from build123d import *

# Parameters (mm, degrees)
SKETCH1_W           = 7
SKETCH1_H           = 7
BOSS_EXTRUDE1_DEPTH = 3
CUT_EXTRUDE1_DEPTH  = 7
CUT_EXTRUDE2_DEPTH  = 11
SKETCH4_R           = 1.8
CUT_EXTRUDE3_DEPTH  = 0.8
CUT_EXTRUDE4_DEPTH  = 0.4


with BuildPart() as part:
    # Sketch1 → Boss-Extrude1 (new body)
    with BuildSketch(Plane(origin=(0, 0, 0), x_dir=(1, 0, 0), z_dir=(0, 1, 0))):
        with Locations((3.5, 3.5)):
            Rectangle(SKETCH1_W, SKETCH1_H)
    extrude(amount=BOSS_EXTRUDE1_DEPTH)

    # Sketch2 → Cut-Extrude1 (cut)
    with BuildSketch(Plane.XY):
        Polygon((0, 0), (0.7, 3), (0, 3), align=None)
        Polygon((7, 0), (6.3, 3), (7, 3), align=None)
    extrude(amount=-CUT_EXTRUDE1_DEPTH, mode=Mode.SUBTRACT)

    # Sketch3 → Cut-Extrude2 (cut)
    with BuildSketch(Plane(origin=(0, 0, 0), x_dir=(0, 0, -1), z_dir=(1, 0, 0))):
        Polygon((0, 0), (0.7, 3), (0, 3), align=None)
        Polygon((7, 3), (6.3, 3), (7, 0), align=None)
    extrude(amount=CUT_EXTRUDE2_DEPTH, mode=Mode.SUBTRACT)

    # Sketch4 → Cut-Extrude3 (cut)
    with BuildSketch(Plane.XZ):
        with Locations(Location((3.5, -3.5, 0), (0, 0, 270))):
            Circle(SKETCH4_R)
    extrude(amount=-CUT_EXTRUDE3_DEPTH, mode=Mode.SUBTRACT)

    # Sketch5 → Cut-Extrude4 (cut)
    with BuildSketch(Plane(origin=(0, 3, 0), x_dir=(1, 0, 0), z_dir=(0, 1, 0))):
        with BuildLine():
            Line((2.046721013, 2.878720245), (2.719797936, 2.92359204))
            add(Edge.make_bspline(
                [(2.719797936, 2.92359204), (2.725160149, 2.895432871), (2.735575908, 2.840735478), (2.758717767, 2.762784225), (2.784190549, 2.69011155), (2.81463192, 2.623496744), (2.847957445, 2.561708471), (2.886904829, 2.506506929), (2.928757004, 2.456129675), (2.975585733, 2.412386043), (3.026605026, 2.374074766), (3.082069463, 2.341401632), (3.14137804, 2.313122445), (3.204675773, 2.289835431), (3.272615043, 2.272451562), (3.344603998, 2.260083969), (3.420745884, 2.252164104), (3.4727828, 2.251073777), (3.499445372, 2.250515117)],
                knots=[0, 0, 0, 0, 1.204560339, 2.339781841, 3.415289417, 4.440034832, 5.416475564, 6.362424008, 7.275913008, 8.16578645, 9.05021719, 9.95355393, 10.867835453, 11.809845306, 12.784702352, 13.812224031, 14.87903166, 16, 16, 16, 16], degree=3))
            add(Edge.make_bspline(
                [(3.499445372, 2.250515117), (3.527509416, 2.250821294), (3.582095427, 2.251416824), (3.661196592, 2.258804896), (3.735159775, 2.269389104), (3.803331854, 2.286143658), (3.866985877, 2.304880975), (3.924540945, 2.330515622), (3.976928433, 2.36008148), (4.024013382, 2.393631069), (4.06510446, 2.430839971), (4.101052986, 2.469684857), (4.132361778, 2.5093265), (4.157004013, 2.551524023), (4.176946643, 2.594570783), (4.190127325, 2.639750939), (4.199031656, 2.686027058), (4.200052723, 2.717653631), (4.200567167, 2.733588033)],
                knots=[0, 0, 0, 0, 1.417779877, 2.757654889, 4.012140507, 5.189587551, 6.302846416, 7.360586765, 8.365575446, 9.33904572, 10.275781718, 11.161696098, 12.012180333, 12.822428111, 13.625933072, 14.403138519, 15.195454004, 16, 16, 16, 16], degree=3))
            add(Edge.make_bspline(
                [(4.200567167, 2.733588033), (4.199936245, 2.753552546), (4.198701939, 2.792610195), (4.183842132, 2.848447381), (4.161557458, 2.900178921), (4.12800444, 2.94704074), (4.082900924, 2.989865612), (4.025366896, 3.029927231), (3.953796381, 3.065967021), (3.900700369, 3.086070082), (3.872442167, 3.096769123)],
                knots=[0, 0, 0, 0, 0.90494901, 1.770400303, 2.607161909, 3.452839393, 4.36912122, 5.420987164, 6.627424851, 8, 8, 8, 8], degree=3))
            add(Edge.make_bspline(
                [(3.872442167, 3.096769123), (3.860317321, 3.100832215), (3.833183883, 3.109924755), (3.786897121, 3.12292623), (3.731143485, 3.139161617), (3.665117302, 3.157615727), (3.588840772, 3.176489423), (3.503165804, 3.199739676), (3.407047926, 3.222875577), (3.339803742, 3.239954494), (3.304533513, 3.248912553)],
                knots=[0, 0, 0, 0, 0.521821638, 1.167752076, 1.961721917, 2.891982557, 3.96540661, 5.168436773, 6.514817513, 8, 8, 8, 8], degree=3))
            add(Edge.make_bspline(
                [(3.304533513, 3.248912553), (3.258601207, 3.260380777), (3.169982333, 3.282506842), (3.043591527, 3.321867543), (2.927183282, 3.360974579), (2.821878423, 3.403407811), (2.726515392, 3.446291426), (2.642636716, 3.492636137), (2.568492031, 3.540035098), (2.525286202, 3.57546224), (2.504553545, 3.592462232)],
                knots=[0, 0, 0, 0, 1.293880989, 2.496331788, 3.617634808, 4.64976062, 5.598842568, 6.473791081, 7.267636666, 8, 8, 8, 8], degree=3))
            add(Edge.make_bspline(
                [(2.504553545, 3.592462232), (2.478842356, 3.616535508), (2.428433193, 3.663733391), (2.362077353, 3.741288571), (2.306320379, 3.82321321), (2.260426285, 3.908902595), (2.225088701, 3.998850035), (2.200041876, 4.092453462), (2.18383066, 4.189957168), (2.182176417, 4.256359502), (2.181336398, 4.290078418)],
                knots=[0, 0, 0, 0, 1.064429417, 2.086912298, 3.078678339, 4.055528992, 5.020032834, 5.993708893, 6.981211098, 8, 8, 8, 8], degree=3))
            add(Edge.make_bspline(
                [(2.181336398, 4.290078418), (2.182972343, 4.333710293), (2.18621757, 4.420262908), (2.215978417, 4.547483438), (2.262337684, 4.670241451), (2.316103441, 4.767715859), (2.367760734, 4.841455617), (2.410658355, 4.894370593), (2.457785536, 4.943893923), (2.509787819, 4.988817578), (2.564734232, 5.031772991), (2.624753609, 5.069917913), (2.688144219, 5.105848319), (2.779877653, 5.148442144), (2.904426487, 5.192829094), (3.06647121, 5.230244475), (3.242905826, 5.252735952), (3.365228488, 5.25549518), (3.428632071, 5.256925373)],
                knots=[0, 0, 0, 0, 1.180131776, 2.341029169, 3.518901375, 4.725685298, 5.343762192, 5.955650671, 6.568945152, 7.192346361, 7.815201106, 8.455999361, 9.116257477, 9.787318263, 11.192748436, 12.688084276, 14.283332633, 16, 16, 16, 16], degree=3))
            add(Edge.make_bspline(
                [(3.428632071, 5.256925373), (3.480546978, 5.25623114), (3.581520363, 5.254880873), (3.727893013, 5.241226755), (3.86461301, 5.219975735), (3.991200587, 5.189469994), (4.107714725, 5.149163904), (4.214607068, 5.10115173), (4.311786782, 5.044149232), (4.3980708, 4.977829293), (4.474941591, 4.904715813), (4.541999061, 4.824854673), (4.599499587, 4.739254471), (4.647814268, 4.647977762), (4.68575566, 4.550555251), (4.713622114, 4.447108501), (4.732053229, 4.337881002), (4.736673044, 4.263037228), (4.739028705, 4.224874091)],
                knots=[0, 0, 0, 0, 1.325124071, 2.577337985, 3.749592149, 4.855247722, 5.896868755, 6.892903601, 7.842551483, 8.766257401, 9.665194363, 10.546067736, 11.423174165, 12.293291263, 13.177512979, 14.086532529, 15.024315359, 16, 16, 16, 16], degree=3))
            Line((4.739028705, 4.224874091), (4.065951782, 4.180002296))
            add(Edge.make_bspline(
                [(4.065951782, 4.180002296), (4.062068972, 4.201108183), (4.054501777, 4.242241362), (4.038048624, 4.301152432), (4.019490266, 4.355638451), (3.997768669, 4.405699072), (3.971531605, 4.45043766), (3.942978139, 4.491261716), (3.911320612, 4.527627281), (3.875510829, 4.55853855), (3.83677937, 4.586666537), (3.792639157, 4.60921177), (3.744939713, 4.630128784), (3.691866364, 4.645853249), (3.634438311, 4.65832646), (3.572622102, 4.667573288), (3.506289601, 4.672088109), (3.460655286, 4.673079253), (3.437045532, 4.67359204)],
                knots=[0, 0, 0, 0, 1.151066407, 2.24330871, 3.278475654, 4.238599069, 5.165719782, 6.056502506, 6.909492653, 7.744782051, 8.590364415, 9.471203867, 10.39832458, 11.382154319, 12.435022857, 13.550631277, 14.73277401, 16, 16, 16, 16], degree=3))
            add(Edge.make_bspline(
                [(3.437045532, 4.67359204), (3.412497837, 4.673139334), (3.364739198, 4.672258574), (3.295142133, 4.666853479), (3.229854863, 4.656876194), (3.168556746, 4.643888244), (3.11132966, 4.626219037), (3.058294374, 4.604674333), (3.009208245, 4.579309585), (2.979277664, 4.559353476), (2.964489443, 4.549493482)],
                knots=[0, 0, 0, 0, 1.186678824, 2.308736671, 3.37120409, 4.377216403, 5.334874112, 6.262130804, 7.141346615, 8, 8, 8, 8], degree=3))
            add(Edge.make_bspline(
                [(2.964489443, 4.549493482), (2.947565565, 4.53602445), (2.914789266, 4.509939115), (2.879515034, 4.458142509), (2.858279864, 4.399639797), (2.855723971, 4.358268553), (2.854413321, 4.337053578)],
                knots=[0, 0, 0, 0, 1.037857257, 2.010007357, 2.979541333, 4, 4, 4, 4], degree=3))
            add(Edge.make_bspline(
                [(2.854413321, 4.337053578), (2.855485194, 4.317226776), (2.857596612, 4.27817113), (2.878892988, 4.22269174), (2.911643913, 4.171286094), (2.942244281, 4.143361874), (2.958179346, 4.128820405)],
                knots=[0, 0, 0, 0, 0.98538058, 1.941042925, 2.927803204, 4, 4, 4, 4], degree=3))
            add(Edge.make_bspline(
                [(2.958179346, 4.128820405), (2.970825874, 4.119382262), (2.9990856, 4.098291942), (3.050851816, 4.07148415), (3.113334997, 4.042449691), (3.187959609, 4.014065302), (3.274229699, 3.985733602), (3.372150512, 3.956152032), (3.481782274, 3.926173301), (3.600330525, 3.897140369), (3.720690389, 3.868602665), (3.835546491, 3.837402899), (3.942346149, 3.806985541), (4.040594163, 3.775103213), (4.130796984, 3.744065866), (4.212516439, 3.712188275), (4.286313644, 3.681143069), (4.372369366, 3.63845371), (4.469904872, 3.580629249), (4.572133086, 3.496571752), (4.662540895, 3.402085635), (4.725534654, 3.312991744), (4.76880807, 3.236368627), (4.796671585, 3.175291081), (4.82077571, 3.110930748), (4.840396402, 3.043216506), (4.854616683, 2.972053072), (4.866384793, 2.897984135), (4.872397339, 2.820394537), (4.873224033, 2.767483952), (4.87364409, 2.740599251)],
                knots=[0, 0, 0, 0, 0.511875881, 1.143829537, 1.88775736, 2.750598373, 3.734912702, 4.837306479, 6.073130119, 7.42648979, 8.801963576, 10.091065733, 11.292408984, 12.408830014, 13.446061236, 14.39066453, 15.257936293, 16.045629259, 17.510392066, 18.929669597, 20.331293837, 21.746891395, 22.460690638, 23.187651344, 23.925159671, 24.69163991, 25.474819891, 26.281170188, 27.126635539, 28, 28, 28, 28], degree=3))
            add(Edge.make_bspline(
                [(4.87364409, 2.740599251), (4.873066499, 2.715805547), (4.871919459, 2.666567652), (4.86390363, 2.593486185), (4.851507352, 2.52170251), (4.833156603, 2.451126638), (4.80881246, 2.381897405), (4.78140289, 2.313015643), (4.747128767, 2.245983517), (4.708120139, 2.18074551), (4.665091851, 2.117350577), (4.616332808, 2.058870196), (4.564706926, 2.003353319), (4.506915449, 1.953908582), (4.44652713, 1.906532418), (4.38077987, 1.864575291), (4.311214031, 1.826607806), (4.237389761, 1.792913428), (4.159045311, 1.763551823), (4.076282436, 1.737417953), (3.988355491, 1.716029388), (3.895997661, 1.697696694), (3.798870959, 1.683755153), (3.697096814, 1.674020716), (3.590652088, 1.66853108), (3.51814807, 1.667637137), (3.481216205, 1.667181783)],
                knots=[0, 0, 0, 0, 0.900570041, 1.788444861, 2.667795364, 3.545012114, 4.433698372, 5.332345486, 6.235991676, 7.164928091, 8.092777575, 9.015680987, 9.928493428, 10.842962589, 11.775229507, 12.714851019, 13.672254427, 14.652424454, 15.660007982, 16.709910502, 17.803296389, 18.945495772, 20.129342395, 21.366102753, 22.658353839, 24, 24, 24, 24], degree=3))
            add(Edge.make_bspline(
                [(3.481216205, 1.667181783), (3.427892291, 1.668052387), (3.324069365, 1.669747473), (3.173233299, 1.684919824), (3.031759055, 1.708142203), (2.899876942, 1.741845708), (2.777425768, 1.785113401), (2.664461381, 1.838409645), (2.561530178, 1.902052856), (2.4673573, 1.97449958), (2.383197452, 2.057069979), (2.307520748, 2.148053225), (2.241348087, 2.248268606), (2.184722964, 2.357559374), (2.136213798, 2.475334702), (2.096207822, 2.601648673), (2.066085424, 2.737103735), (2.053287453, 2.830698323), (2.046721013, 2.878720245)],
                knots=[0, 0, 0, 0, 1.217954099, 2.371385517, 3.459848295, 4.490682126, 5.476952527, 6.422732854, 7.338496285, 8.236688651, 9.131557988, 10.026443255, 10.935708282, 11.869506048, 12.834296687, 13.842423496, 14.892981177, 16, 16, 16, 16], degree=3))
        make_face()
    extrude(amount=-CUT_EXTRUDE4_DEPTH, mode=Mode.SUBTRACT)


solid = part.part
Source: CAD feature listing. Evaluate the final solid. Frame: model axes, mm. A direction names the side the tool comes from. Round coordinates to 2 decimals unless told otherwise and drop trailing zeros. Loops run counter-clockwise (first coordinate to the right, second up) from the corner with the lowest first, then second, coordinate; pieces in that order, holes last. Notation, with made-up numbers: (68.5, 87) - (109.5, 87) arc R9 cw to (109.5, 99) - close; hole circle Ø6 at (53.5, -39.5). An arc over 180 degrees is marked (long way). Write item = value, one per line. Start each with the question number.
Item 1: First-contact query: pin 1 Ø1.5 at (y, z) = (1, -1.5) entering from +X. Flat tip, straight axial feed; report the tip coordinate or a pass-through.
Item 2: Section query B-B on x = 1.25. Output: boundary loops of the cut face in (y, z), plus the area to 3 significant figures.
Item 3: Section query D-D on x = 5. Output: boundary loops of the cut face in (y, z), plus the area to 3 significant figures.
Item 4: Section query C-C on y = 1.25. Output: boundary loops of the cut face in (x, z).
Item 5: Material intervals for line 1 (Y direction, x = 2.25, z = -2.5); line 2 (Y direction, x = 2, z = -3.25); line 3 (Z direction, x = 5.75, y = 2.9), sorted ascending.
Item 6: Reachability of faces 1 (the face through (4.041, 0.394, -5.217)), 2 (the face through (3.5, 3, -4.2)) from +Z, -Z, +X, -X, +Y, -Y: full face, straight path, thin tool, end or side. Return the list, or none.
Item 7: Mould query, pull axis X, two halves, no side actions, for faces 3 (the face through (3.5, 2.6, -3.5)), 4 (the face through (4, 0.8, -3)), 5 (the face through (6.655, 1.479, -3.451)), 6 (the face through (3.451, 1.521, -6.645)). Classes: released by +X, released by -X, zero draft, split by the parting line, or undercut.
Item 8: Section query A-A on y = 0.3. Output: boundary loops of the cut face in (x, z).
Results list:
q1.pin_1 = 6.94
q2.outline = (0, -7) - (3, -6.3) - (3, -0.7) - (0, 0) - close
q2.area = 18.9 mm²
q3.outline = (0, -7) - (3, -6.3) - (3, -0.7) - (0, 0) - (0, -2.51) - (0.8, -2.51) - (0.8, -4.49) - (0, -4.49) - close
q3.area = 17.3 mm²
q4.outline = (0.29, -6.71) - (6.71, -6.71) - (6.71, -0.29) - (0.29, -0.29) - close
q5.line_1 = 0.8 to 2.6
q5.line_2 = 0.8 to 3
q5.line_3 = -6.32 to -0.68
q6.face_1 = -Y
q6.face_2 = +Z, -Z, +X, -X, +Y
q7.face_3 = undercut
q7.face_4 = undercut
q7.face_5 = released by +X
q7.face_6 = zero draft
q8.outline = (0.07, -6.93) - (6.93, -6.93) - (6.93, -0.07) - (0.07, -0.07) - close; hole circle Ø3.6 at (3.5, -3.5)
